Source: CAD feature listing. Evaluate the final solid. Frame: model axes, mm. Give positions to 0.01 mm unless a question says otherwise; leave off trailing zeros. Loops run counter-clockwise (first coordinate to the right, second up) from the corner with the lowest first, then second, coordinate; pieces in that order, holes last. Notation, with made-up numbers: (89.5, 82) -> (138.5, 82) arc R15 cw to (138.5, 105) -> close; hole circle Ø2 at (19.25, 75). An arc over 180 degrees is marked (long way). Return JSON: item names as keys, results as strings. Group by question number.
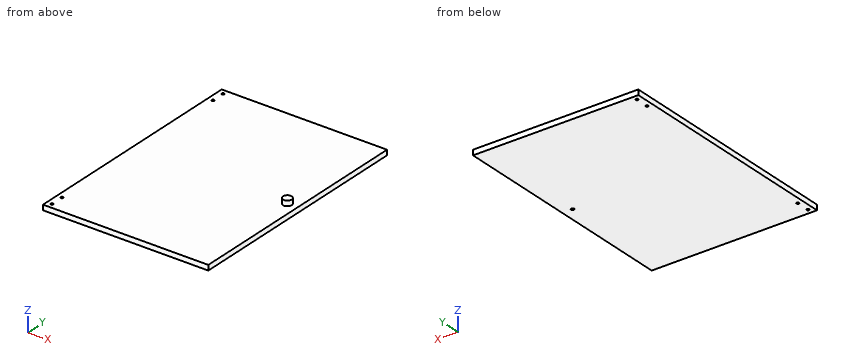
```python
from build123d import *

# Parameters (mm, degrees)
SKETCH1_W           = 320
SKETCH1_H           = 460
SKETCH1_R           = 2.5
SKETCH1_R_2         = 3
BOSS_EXTRUDE1_DEPTH = 10
SKETCH2_R           = 8.578403593
BOSS_EXTRUDE2_DEPTH = 10


with BuildPart() as part:
    # Sketch1 → Boss-Extrude1 (new body)
    with BuildSketch(Plane.XY):
        Rectangle(SKETCH1_W, SKETCH1_H)
        with Locations((-150, -220)):
            Circle(SKETCH1_R, mode=Mode.SUBTRACT)
        with Locations((-150, 220)):
            Circle(SKETCH1_R, mode=Mode.SUBTRACT)
        with Locations((140, 0)):
            Circle(SKETCH1_R_2, mode=Mode.SUBTRACT)
        with Locations((-150, -194)):
            Circle(SKETCH1_R, mode=Mode.SUBTRACT)
        with Locations((-150, 194)):
            Circle(SKETCH1_R, mode=Mode.SUBTRACT)
    extrude(amount=BOSS_EXTRUDE1_DEPTH)

    # Sketch2 → Boss-Extrude2 (add)
    with BuildSketch(Plane.XY.offset(10)):
        with Locations((140, 0)):
            Circle(SKETCH2_R)
    extrude(amount=BOSS_EXTRUDE2_DEPTH)


solid = part.part
```
1) Cut plane C-C on y = -73. Return loops of the section in (x, z).
2) Cut plane A-A on x = -94.5. Return loops of the section in (y, z), then the cut area to 3 significant figures.
3) Cut plane B-B on z = 16.75. Return loops of the section in (x, y), then the cut area to 3 significant figures.
4) Material intervals for line 1 (Y direction, x = -150, z = 3.25); line 2 (Y direction, x = 140, z = 2.75); line 3 (X direction, y = -220, z = 3.75), sorted ascending.
5) Contact query for flat-ended pins moving along their axis: P1, Ø1, axis at x = -105, y = -133, coming from the +Z side; P2, Ø5.5, axis at x = 140, y = 0, coming from the -Z side. Output: stop coordinate, or through.
Calculated:
{
 "1": {"outline": "(-160, 0) -> (160, 0) -> (160, 10) -> (-160, 10) -> close"},
 "2": {"outline": "(-230, 0) -> (230, 0) -> (230, 10) -> (-230, 10) -> close", "area": "4,600 mm2"},
 "3": {"outline": "circle Ø17.16 at (140, 0)", "area": "231 mm2"},
 "4": {"line 1": "-230 to -222.5, -217.5 to -196.5, -191.5 to 191.5, 196.5 to 217.5, 222.5 to 230", "line 2": "-230 to -3, 3 to 230", "line 3": "-160 to -152.5, -147.5 to 160"},
 "5": {"P1": "z = 10", "P2": "z = 10"}
}
